Source: CAD feature listing. Evaluate the final solid. Frame: model axes, mm. Give positions to 0.01 mm unless a question says otherwise; leave off trailing zeros. Use CSV: the item, a comma, the result in double quotes. Start each with the question number.
Autodesk Inventor part; units mm, degrees
ref_plane "YZ Plane" through (0, 0, 0) normal (1, 0, 0) x (0, 1, 0)
ref_plane "XZ Plane" through (0, 0, 0) normal (0, 1, 0) x (-1, 0, 0)
ref_plane "XY Plane" through (0, 0, 0) normal (0, 0, 1) x (1, 0, 0)
sketch "Sketch3" plane through (0, 0, 0) normal (0, 1, 0) x (-1, 0, 0)
  line L0 (0, 0) -> (-152.4, 0)
  line L1 (-152.4, 0) -> (-152.4, -215.9)
  line L2 (-152.4, -215.9) -> (0, -215.9)
  line L3 (0, -215.9) -> (0, 0)
  dimension "d8" = 152.4
  dimension "d9" = 215.9
extrude "Extrusion1" add sketch "Sketch3" against normal blind 3.175
sketch "Sketch4" plane through (0, 0, 0) normal (0, 1, 0) x (1, 0, 0)
  line L0 (152.4, 0) -> (152.4, 215.9)
  line L1 (0, 0) -> (152.4, 0)
  line L2 (152.4, 215.9) -> (0, 215.9)
  point P0 (126.3904, 63.0378)
  point P1 (126.3904, 148.7849)
  point P2 (73.406, 188.5442)
  point P3 (73.406, 27.3558)
  dimension "d12" = 26.0096
  dimension "d13" = 26.0096
  dimension "d14" = 78.994
  dimension "d15" = 78.994
  dimension "d16" = 27.3558
  dimension "d17" = 27.3558
  dimension "d29" = 63.0378
  dimension "d30" = 67.1151
hole "Hole1" at (126.3904, 0, -63.0378) at (126.3904, 0, -148.7849) at (73.406, 0, -188.5442) at (73.406, 0, -27.3558) direction (0, -1, 0) diameter 5.9944 end through all
sketch "Sketch5" plane through (0, 0, 0) normal (0, 1, 0) x (1, 0, 0)
  circle A0 centre (126.3904, 148.7849) radius 2.9972
  circle A1 centre (126.3904, 148.7849) radius 6.477
  circle A2 centre (126.3904, 63.0378) radius 2.9972
  circle A3 centre (126.3904, 63.0378) radius 6.477
  circle A4 centre (73.406, 27.3558) radius 2.9972
  circle A5 centre (73.406, 27.3558) radius 10.9855
  circle A6 centre (73.406, 188.5442) radius 2.9972
  circle A7 centre (73.406, 188.5442) radius 10.9855
  line L0 (131.1992, 58.6988) -> (80.1831, 18.7099)
  line L1 (132.8674, 63.0378) -> (132.8674, 148.7849)
  line L2 (80.1831, 197.1901) -> (129.3876, 154.5267)
  line L3 (62.4205, 27.3558) -> (62.4205, 188.5442)
  point P0 (0, 0)
  dimension "d25" = 12.954
  dimension "d26" = 12.954
  dimension "d27" = 21.971
  dimension "d28" = 21.971
properties part number "recreated v of plate"
1. Line query: probe 1 along X at (y, z) = (-2.15, -191); probe 2 along X at (y, z) = (-2, -151). Output: solid intervals per line, ascending.
2. First-contact query: pin 1 (3.5 mm diameter, centred on x = 73.41, z = -188.54, fed in from +Y). Flat tip, straight axial feed; report the tip coordinate or a pass-through.
3. Pull-direction query (X, two-part tool) for faces 1 (the cylindrical face through (129.05, -1.61, -147.4)), 2 (the flat face through (77, 0, -106)); classes: released by +X, released by -X, zero draft, split by the parting line, or undercut.
Resolved:
1,probe 1,"x = 0 to 71.69, 75.12 to 152.4"
1,probe 2,"x = 0 to 124.37, 128.41 to 152.4"
2,pin 1,"passes through"
3,face 1,"undercut"
3,face 2,"zero draft"
